Here's how the part is built. I have some questions about the finished solid (model axes, mm). Round coordinates to 2 decimals unless told otherwise and drop trailing zeros. Loops run counter-clockwise (first coordinate to the right, second up) from the corner with the lowest first, then second, coordinate; pieces in that order, holes last. Notation, with made-up numbers: M 49,83.25 L 67,83.25 A28 cw 67,121.25 Z; hole C -16.75,-8 d7. An arc over 180 degrees is marked long. Answer as a JSON object with one key per item and string values.
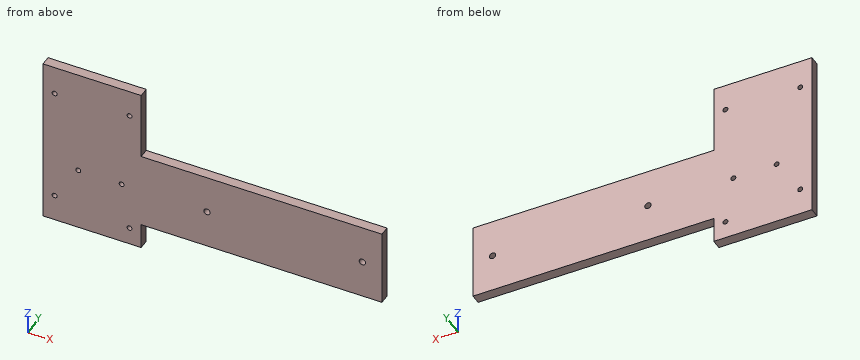
from build123d import *

# Parameters (mm, degrees)
SKETCH1_W           = 63.2
SKETCH1_H           = 111.6
SKETCH1_W_2         = 53.2
SKETCH1_H_2         = 101.6
SKETCH1_R           = 1.6
BOSS_EXTRUDE1_DEPTH = 6.35
SKETCH2_W           = 155
SKETCH2_H           = 50
SKETCH2_R           = 2.05
BOSS_EXTRUDE2_DEPTH = 6.35


with BuildPart() as part:
    # Sketch1 → Boss-Extrude1 (new body)
    # profile 1 of 2: a face of its own
    with BuildSketch(Plane(origin=(0, 0, 0), x_dir=(1, 0, 0), z_dir=(0, 1, 0))):
        with Locations((-26.6, 50.8)):
            Rectangle(SKETCH1_W, SKETCH1_H)
        with Locations((-26.6, 50.8)):
            Rectangle(SKETCH1_W_2, SKETCH1_H_2, mode=Mode.SUBTRACT)
    # profile 2 of 2: a face of its own
    with BuildSketch(Plane(origin=(0, 0, 0), x_dir=(1, 0, 0), z_dir=(0, 1, 0))):
        with Locations((-26.6, 50.8)):
            Rectangle(SKETCH1_W_2, SKETCH1_H_2)
        with Locations(Location((-2.5, 12.7, 0), (0, 0, 270))):
            Circle(SKETCH1_R, mode=Mode.SUBTRACT)
        with Locations(Location((-50.7, 14, 0), (0, 0, 270))):
            Circle(SKETCH1_R, mode=Mode.SUBTRACT)
        with Locations(Location((-7.6, 64.8, 0), (0, 0, 270))):
            Circle(SKETCH1_R, mode=Mode.SUBTRACT)
        with Locations(Location((-35.5, 64.8, 0), (0, 0, 270))):
            Circle(SKETCH1_R, mode=Mode.SUBTRACT)
        with Locations(Location((-2.5, 95.05, 0), (0, 0, 270))):
            Circle(SKETCH1_R, mode=Mode.SUBTRACT)
        with Locations(Location((-50.7, 88.9, 0), (0, 0, 270))):
            Circle(SKETCH1_R, mode=Mode.SUBTRACT)
    extrude(amount=BOSS_EXTRUDE1_DEPTH)

    # Sketch2 → Boss-Extrude2 (add)
    with BuildSketch(Plane(origin=(0, 6.35, 0), x_dir=(1, 0, 0), z_dir=(0, 1, 0))):
        with Locations((82.5, 64.8)):
            Rectangle(SKETCH2_W, SKETCH2_H)
        with Locations(Location((47.4, 64.8, 0), (0, 0, 270))):
            Circle(SKETCH2_R, mode=Mode.SUBTRACT)
        with Locations(Location((147.4, 64.8, 0), (0, 0, 270))):
            Circle(SKETCH2_R, mode=Mode.SUBTRACT)
    extrude(amount=-BOSS_EXTRUDE2_DEPTH)


solid = part.part
Item 1: I want a section at A-A on x = 47.4. List the corners of the cut face in (y, z) for me.
Solution:
{"outline": "M 0,-89.8 L 6.35,-89.8 L 6.35,-66.85 L 0,-66.85 Z; M 0,-62.75 L 6.35,-62.75 L 6.35,-39.8 L 0,-39.8 Z"}
Item 2: I want a section at D-D on x = 22.5. List the corners of the cut face in (y, z) for me, plus the area to 4 significant figures.
Solution:
{"outline": "M 0,-89.8 L 6.35,-89.8 L 6.35,-39.8 L 0,-39.8 Z", "area": "317.5 mm2"}
Item 3: For P1, Ø1.9, axis at y = 4.5, z = -28.5, coming from the +X side; P2, Ø1.9, axis at x = -2.5, z = -12.7, coming from the -Y side; P3, Ø1.9, axis at x = 62, y = 2.5, coming from the +Z side, each with a flat end and sliding along its axis, tell me the tip position at first contact or that it passes through.
Solution:
{"P1": "stops at x = 5", "P2": "passes through", "P3": "stops at z = -39.8"}
Item 4: If I drill on L1, parallel to X at y = 3, z = -64.8; L2, parallel to X at y = 3, z = -13; L3, parallel to X at y = 4, z = -12.7, over which ranges is the centre line in solid material (lowest first)? Write a range as from..to.
Solution:
{"L1": "x = -58.2..-37.1, -33.9..-9.2, -6..45.35, 49.45..145.35, 149.45..160", "L2": "x = -58.2..-51.95, -49.45..-4.07, -0.93..5", "L3": "x = -58.2..-51.63, -49.77..-4.1, -0.9..5"}
Item 5: I want a section at C-C on z = -3. List the corners of the cut face in (x, y) for me.
Solution:
{"outline": "M -58.2,0 L 5,0 L 5,6.35 L -58.2,6.35 Z"}
Item 6: I want a section at B-B on y = 4.75. Count the separate pieces of the cut face and the enclosed holes in it, plus the area to 3 significant figures.
Solution:
{"separate pieces": "1", "enclosed holes": "8", "area": "14,700 mm2"}
